Work out the finished part from the listing and answer in its coordinate system (mm). A direction names the side the tool comes from. Coordinates: 2 decimals unless noted, no trailing zeros. Order: outer loops, then holes, each group sorted by start corner. A loop starts at its lowest first (then second) coordinate and runs counter-clockwise, first axis right, second up. Notation, with made-up numbers: M 60,9 L 107,9 A14 ccw 107,23 Z; hole C -29,-27 d2. An arc over 180 degrees is marked long. Answer in a Markdown table with one row per item. Add a question column.
Item 1: The part is cut by section C-C (z = -22.5). Write down the section's boundary in (x, y), then the cut area to 3 significant figures.
Item 2: The part is cut by section A-A (x = -49). Write down the section's boundary in (y, z), then the cut area to 3 significant figures.
Item 3: Flat-ended cylindrical pins translate along their axes: pin 1 Ø8 at (x, y) = (-13.5, 15.5) entering from +Z; pin 2 Ø2 at (y, z) = (-8.5, -13.5) entering from -X; pin 3 Ø2 at (x, y) = (-53.5, 10) entering from +Z; pin 4 Ø10 at (x, y) = (12.7, 19.05) entering from +Z. Find the tip coordinate at first contact, or state that the pin passes through.
Item 4: Consider line 1 (Y direction, x = 16, z = -11); line 2 (Z direction, x = 14, y = -10); line 3 (X direction, y = -5, z = -14). Determine where each line is inside the solid, lowest interval first. Write a range as from..to.
Item 5: The part is cut by section D-D (z = -14). Write down the section's boundary in (x, y).
Item 6: The mould has two halves that part along X. Classify faces 1 (the face through (18.006, -17.379, -10.181)), 2 (the face through (-62.245, -0.444, -59.924)), 3 (the face through (-21, 31.75, -29)), 4 (the face through (58.75, -0.19, -10.18)): released by +X, released by -X, zero draft, split by the parting line, or undercut.
Item 7: Which of the six approach directions +Z, -Z, +X, -X, +Y, -Y give full straight-line access (tool end or side, diameter ignored) to faces 5 (the face through (11.734, -31.713, -3.297)), 6 (the face through (22, -7, -20.65)), 7 (the face through (-7.31, -18.45, -24.07)), 8 (the face through (-7.31, 18.07, -24.07))?
Item 8: The part is cut by section B-B (y = 0). Write down the section's boundary in (x, z), then the cut area to 3 significant figures.
from build123d import *

# Parameters (mm, degrees)
F0_R     = 5.5626
F1_DEPTH = 20.6502
F2_R     = 19.05
F3_DEPTH = 31.75
F5_DEPTH = 4.7625
F6_R     = 5.5626
F7_DEPTH = 68.2762


with BuildPart() as f1:
    # F0 (on Top) → F1 (new body)
    with BuildSketch(Plane.XY):
        with BuildLine():
            ThreePointArc((18.9991554441, 30.0777214642), (6.3246284085, 30.0338352623), (0, 19.05))
            Line((0, 19.05), (0, -19.05))
            ThreePointArc((0, -19.05), (6.3246284085, -30.0338352623), (18.9991554441, -30.0777214642))
            Line((18.9991554441, -30.0777214642), (52.3493554441, -11.0277214642))
            ThreePointArc((52.3493554441, -11.0277214642), (58.7502, 0), (52.3493554441, 11.0277214642))
            Line((52.3493554441, 11.0277214642), (18.9991554441, 30.0777214642))
        make_face()
        with Locations((12.7, -19.05)):
            Circle(F0_R, mode=Mode.SUBTRACT)
        with Locations((12.7, 19.05)):
            Circle(F0_R, mode=Mode.SUBTRACT)
        with Locations((46.0502, 0)):
            Circle(F0_R, mode=Mode.SUBTRACT)
    extrude(amount=-F1_DEPTH)

    # F2 (on Front) → F3 (join, symmetric)
    with BuildSketch(Plane.XZ):
        with BuildLine():
            Line((12.7, -4.7752), (-40.7836134373, -4.7752))
            ThreePointArc((-40.7836134373, -4.7752), (-61.4351988672, -60.6410561787), (-9.4116031009, -31.6405846154))
            ThreePointArc((-9.4116031009, -31.6405846154), (-7.2347568536, -23.979724371), (0, -20.6502))
            Line((0, -20.6502), (12.7, -20.6502))
            Line((12.7, -20.6502), (12.7, -4.7752))
        make_face()
        with Locations((-40.7836134373, -36.5252)):
            Circle(F2_R, mode=Mode.SUBTRACT)
    extrude(amount=F3_DEPTH, both=True)

    # F4 (on Front) → F5 (join, symmetric)
    with BuildSketch(Plane.XZ):
        with BuildLine():
            ThreePointArc((-9.4116031009, -31.6405846154), (-11.1459036377, -47.9124146654), (-20.7531221582, -61.1593616281))
            Line((-20.7531221582, -61.1593616281), (29.0663865627, -20.6502))
            Line((29.0663865627, -20.6502), (0, -20.6502))
            ThreePointArc((0, -20.6502), (-7.2347568536, -23.979724371), (-9.4116031009, -31.6405846154))
        make_face()
    extrude(amount=F5_DEPTH, both=True)

    # F6 (on face) → F7 (cut, through all)
    with BuildSketch(Plane.XY):
        with Locations((12.7, -19.05)):
            Circle(F6_R)
        with Locations((12.7, 19.05)):
            Circle(F6_R)
    extrude(amount=-F7_DEPTH, mode=Mode.SUBTRACT)


solid = f1.part
Reply:
| question | item | result |
|---|---|---|
| 1 | outline | M -69.27,-31.75 L -53.68,-31.75 L -53.68,31.75 L -69.27,31.75 Z; M -27.89,-31.75 L -5.64,-31.75 L -5.64,-4.76 L 26.79,-4.76 L 26.79,4.76 L -5.64,4.76 L -5.64,31.75 L -27.89,31.75 Z |
| 1 | area | 2,710 mm2 |
| 2 | outline | M -31.75,-67.19 L 31.75,-67.19 L 31.75,-53.71 L -31.75,-53.71 Z; M -31.75,-19.34 L 31.75,-19.34 L 31.75,-5.86 L -31.75,-5.86 Z |
| 2 | area | 1,710 mm2 |
| 3 | pin 1 | stops at z = -4.78 |
| 3 | pin 2 | stops at x = -63.65 |
| 3 | pin 3 | stops at z = -7.02 |
| 3 | pin 4 | passes through |
| 4 | line 1 | y = -31.31..-23.53, -14.57..14.57, 23.53..31.31 |
| 4 | line 2 | z = -20.65..0 |
| 4 | line 3 | x = -63.16..43.61, 48.49..57.72 |
| 5 | outline | M -63.16,-31.75 L 12.7,-31.75 A12.7 ccw 19,-30.08 L 52.35,-11.03 A12.7 ccw 52.35,11.03 L 19,30.08 A12.7 ccw 12.7,31.75 L -63.16,31.75 Z; hole C 12.7,-19.05 d11.13; hole C 12.7,19.05 d11.13; hole C 46.05,0 d11.13 |
| 6 | face 1 | undercut |
| 6 | face 2 | split by the parting line |
| 6 | face 3 | zero draft |
| 6 | face 4 | released by +X |
| 7 | face 5 | +Z, -Y |
| 7 | face 6 | -Z, +X |
| 7 | face 7 | +X, -Y |
| 7 | face 8 | +X, +Y |
| 8 | outline | M -40.78,-4.78 A31.75 ccw long -20.75,-61.16 L 29.07,-20.65 L 40.49,-20.65 L 40.49,0 L 0,0 L 0,-4.78 Z; M 51.61,-20.65 L 58.75,-20.65 L 58.75,0 L 51.61,0 Z; hole C -40.78,-36.53 d38.1 |
| 8 | area | 3,990 mm2 |
